Autodesk Inventor part; units mm, degrees
ref_plane "YZ Plane" through (0, 0, 0) normal (1, 0, 0) x (0, 1, 0)
ref_plane "XZ Plane" through (0, 0, 0) normal (0, 1, 0) x (-1, 0, 0)
ref_plane "XY Plane" through (0, 0, 0) normal (0, 0, 1) x (1, 0, 0)
sketch "Sketch1" plane through (0, 0, 0) normal (0, 1, 0) x (-1, 0, 0)
  line L0 (0, 0) -> (-81, 0)
  line L1 (6, -23.0013) -> (13, -30.0013)
  line L2 (13, -30.0013) -> (13, -44.4987)
  line L3 (13, -44.4987) -> (2.7487, -54.75)
  line L4 (2.7487, -54.75) -> (-11.7487, -54.75)
  line L5 (-11.7487, -54.75) -> (-22, -44.4987)
  line L6 (-22, -44.4987) -> (-22, -30.0013)
  line L7 (-59, -30.0013) -> (-59, -44.4987)
  line L8 (-59, -44.4987) -> (-69.2513, -54.75)
  line L9 (-69.2513, -54.75) -> (-83.7487, -54.75)
  line L10 (-83.7487, -54.75) -> (-94, -44.4987)
  line L11 (-94, -44.4987) -> (-94, -30.0013)
  line L12 (-94, -30.0013) -> (-87, -23.0013)
  line L13 (-4.5, -37.25) -> (-76.5, -37.25) construction
  line L14 (-8.6421, -27.25) -> (-0.3579, -27.25)
  line L15 (-0.3579, -27.25) -> (5.5, -33.1079)
  line L16 (5.5, -33.1079) -> (5.5, -41.3921)
  line L17 (5.5, -41.3921) -> (-0.3579, -47.25)
  line L18 (-0.3579, -47.25) -> (-8.6421, -47.25)
  line L19 (-8.6421, -47.25) -> (-14.5, -41.3921)
  line L20 (-14.5, -41.3921) -> (-14.5, -33.1079)
  line L21 (-14.5, -33.1079) -> (-8.6421, -27.25)
  line L22 (-80.6421, -27.25) -> (-72.3579, -27.25)
  line L23 (-72.3579, -27.25) -> (-66.5, -33.1079)
  line L24 (-66.5, -33.1079) -> (-66.5, -41.3921)
  line L25 (-66.5, -41.3921) -> (-72.3579, -47.25)
  line L26 (-72.3579, -47.25) -> (-80.6421, -47.25)
  line L27 (-80.6421, -47.25) -> (-86.5, -41.3921)
  line L28 (-86.5, -41.3921) -> (-86.5, -33.1079)
  line L29 (-86.5, -33.1079) -> (-80.6421, -27.25)
  line L30 (6, -23.0013) -> (6, -6)
  line L31 (6, -6) -> (0, 0)
  line L32 (-81, 0) -> (-87, -6)
  line L33 (-87, -6) -> (-87, -23.0013)
  line L34 (-22, -30.0013) -> (-27.0013, -25)
  line L35 (-27.0013, -25) -> (-53.9987, -25)
  line L36 (-53.9987, -25) -> (-59, -30.0013)
  point P0 (-40.5, -37.25)
  point P1 (-40.5, 0)
  dimension "d0" = 81
  dimension "d1" = 37.25
  dimension "d2" = 72
  dimension "d3" = 20
  dimension "d4" = 20
  dimension "d5" = 45
  dimension "d6" = 6
  dimension "d7" = 35
  dimension "d8" = 35
  dimension "d17" = 7
  dimension "d20" = 45
  dimension "d21" = 25
extrude "Extrusion1" add sketch "Sketch1" along normal blind 6.5
sketch "Sketch2" plane through (0, 6.5, 0) normal (0, 1, 0) x (1, 0, 0)
  line L0 (0, 0) -> (81, 0)
  line L1 (38.25, 16.3) -> (42.75, 16.3)
  line L2 (42.75, 0) -> (38.25, 0)
  line L3 (45.25, 12.3) -> (45.25, 5)
  line L4 (35.75, 5) -> (35.75, 12.3)
  line L5 (38.25, 0) -> (38.25, 5)
  line L6 (38.25, 12.3) -> (38.25, 16.3)
  line L7 (42.75, 16.3) -> (42.75, 12.3)
  line L8 (42.75, 5) -> (42.75, 0)
  line L9 (35.75, 12.3) -> (38.25, 12.3)
  line L10 (42.75, 12.3) -> (45.25, 12.3)
  line L11 (45.25, 5) -> (42.75, 5)
  line L12 (38.25, 5) -> (35.75, 5)
  point P0 (40.5, 0)
  dimension "d24" = 4.5
  dimension "d25" = 4
  dimension "d26" = 5
  dimension "d27" = 7.3
  dimension "d28" = 2.5
extrude "Extrusion2" cut sketch "Sketch2" against normal through all
sketch "Sketch3" plane through (0, 6.5, 0) normal (0, 1, 0) x (1, 0, 0)
  line L0 (42.75, 0) -> (81, 0)
  line L1 (0, 0) -> (38.25, 0)
  line L2 (38.25, 16.3) -> (42.75, 16.3)
  line L3 (15, 0) -> (23, 0)
  line L4 (23, 0) -> (23, -4.5)
  line L5 (21, -6.5) -> (17, -6.5)
  line L6 (15, -4.5) -> (15, 0)
  line L7 (58, 0) -> (66, 0)
  line L8 (66, 0) -> (66, -4.5)
  line L9 (64, -6.5) -> (60, -6.5)
  line L10 (58, -4.5) -> (58, 0)
  arc A0 (15, -4.5) -> (17, -6.5) centre (17, -4.5) ccw
  arc A1 (21, -6.5) -> (23, -4.5) centre (21, -4.5) ccw
  arc A2 (58, -4.5) -> (60, -6.5) centre (60, -4.5) ccw
  arc A3 (64, -6.5) -> (66, -4.5) centre (64, -4.5) ccw
  point P0 (40.5, 16.3)
  dimension "d31" = 2
  dimension "d32" = 8
  dimension "d33" = 8
  dimension "d34" = 6.5
  dimension "d35" = 35
  dimension "d36" = 17.5
extrude "Extrusion3" add sketch "Sketch3" against normal blind 6.5
sketch "Sketch4" plane through (0, 6.5, 0) normal (0, 1, 0) x (1, 0, 0)
  line L0 (66, -4.5) -> (66, 0)
  line L1 (66, 0) -> (81, 0)
  line L2 (73, 5.7735) -> (78, 2.8868)
  line L3 (78, 2.8868) -> (78, 0)
  line L4 (68, 0) -> (68, 2.8868)
  line L5 (68, 2.8868) -> (73, 5.7735)
  line L6 (78, 0) -> (68, 0)
  point P0 (73, 0)
  dimension "d39" = 10
  dimension "d40" = 2
extrude "Extrusion4" cut sketch "Sketch4" against normal through all
equation "\"d33\" = d32"
properties part number "filament_guide" material "Plywood, Finish"
Build history of the part. All positions in model axes, mm. A direction names the side the tool comes from. Round coordinates to 2 decimals unless told otherwise and drop trailing zeros. Loops run counter-clockwise (first coordinate to the right, second up) from the corner with the lowest first, then second, coordinate; pieces in that order, holes last.
Item 1: Pin check, flat tips, straight feed: P1, Ø0.9, axis at y = 2, z = -1, coming from the -X side; P2, Ø0.9, axis at x = 79, y = 1.5, coming from the +Z side; P3, Ø2, axis at y = 2, z = -24, coming from the -X side. Stop position of each tip, or through.
Item 2: Saw through at D-D (y = 2.5). State how many separate pieces and enclosed holes the cut face has, then the cut area to 3 significant figures.
Item 3: Saw through at A-A (z = -40). List the corners of the cut face in (x, y), then the cut area to 3 significant figures.
Item 4: Two-plate mould, pull along Z, no slides. Class faces 5 (the face through (79, 3, 0)), 6 (the face through (38.25, 3, -14)), 7 (the face through (4, 3, -54.75)), 8 (the face through (66.5, 3, -37)): released by +Z, released by -Z, zero draft, split by the parting line, or undercut.
Item 5: Which spindle directions (+Z, -Z, +X, -X, +Y, -Y) get a long thin tool onto all of the face, cutting with end or side? Do faces 1 (the face through (65.4, 3.3, 5.93)), 2 (the face through (44, 3, -12.3)), 3 (the face through (70.465, 3.296, -4.31)), 4 (the face through (22, 3, -37)). Say none if no direction does.
Item 6: Saw through at B-B (z = 2.5). List the corners of the cut face in (x, y).
Item 7: Saw through at C-C (z = -4). List the corners of the cut face in (x, y).
Item 8: Drill centre lines: line 1 along X through (y, z) = (2.5, -40.5); line 2 along Z through (x, y) = (7.5, 5.75); line 3 along Z through (x, y) = (44, 1). Where is each one in solid material? Low to high.
Worked answers:
1. P1: stops at x = -1.45
1. P2: stops at z = 0
1. P3: stops at x = -8
2. separate pieces: 1
2. enclosed holes: 2
2. area: 3,450 mm2
3. outline: (-13, 0) - (-5.5, 0) - (-5.5, 6.5) - (-13, 6.5) - close; (14.5, 0) - (22, 0) - (22, 6.5) - (14.5, 6.5) - close; (59, 0) - (66.5, 0) - (66.5, 6.5) - (59, 6.5) - close; (86.5, 0) - (94, 0) - (94, 6.5) - (86.5, 6.5) - close
3. area: 195 mm2
4. face 5: released by +Z
4. face 6: zero draft
4. face 7: released by -Z
4. face 8: undercut
5. face 1: +Z, +X, +Y, -Y
5. face 2: +Y, -Y
5. face 3: +Z, +Y, -Y
5. face 4: -Z, +Y, -Y
6. outline: (15, 0) - (23, 0) - (23, 6.5) - (15, 6.5) - close; (58, 0) - (66, 0) - (66, 6.5) - (58, 6.5) - close
7. outline: (-4, 0) - (38.25, 0) - (38.25, 6.5) - (-4, 6.5) - close; (42.75, 0) - (69.93, 0) - (69.93, 6.5) - (42.75, 6.5) - close; (76.07, 0) - (85, 0) - (85, 6.5) - (76.07, 6.5) - close
8. line 1: x = -13 to -5.5, 14.5 to 22, 59 to 66.5, 86.5 to 94
8. line 2: z = -54.75 to -47.25, -27.25 to 0
8. line 3: z = -25 to -12.3, -5 to 0
